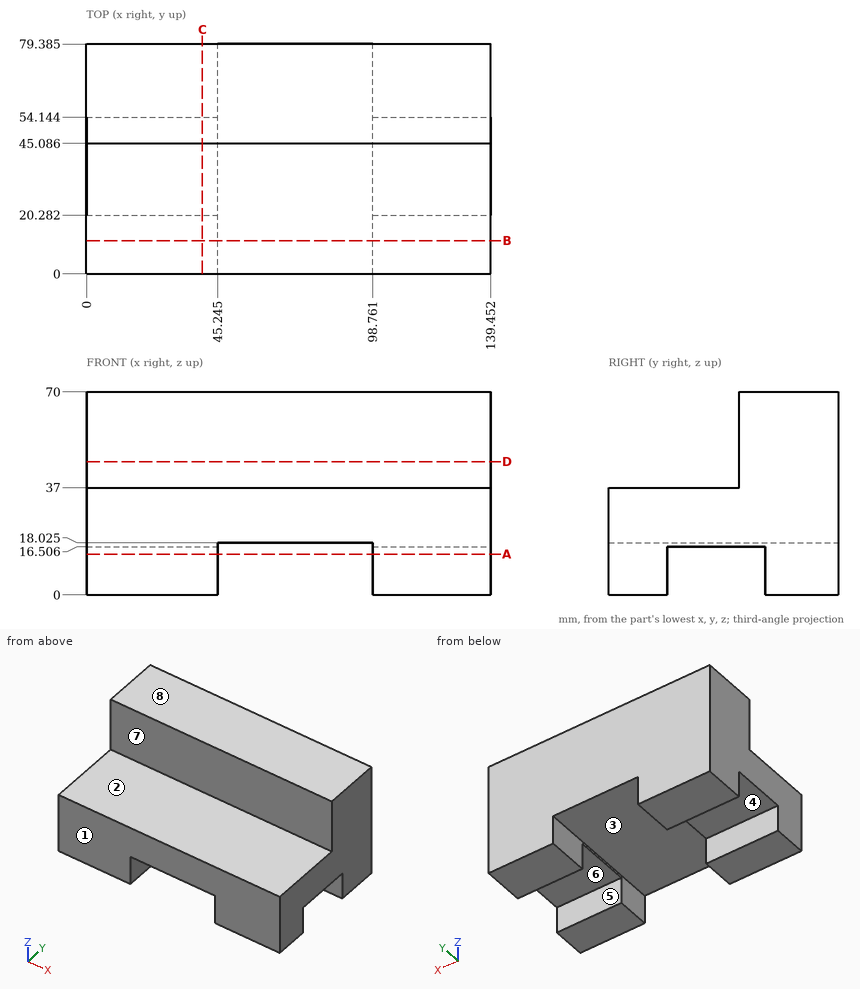
Drawing for the job (mm, zero at the part's lowest x, y, z). A direction names the side the tool comes from. Coordinates: 2 decimals unless noted, no trailing zeros. Write each loop counter-clockwise with the first axis right and the second up, starting at its lowest first coordinate (ties: lowest second). Pieces come first, ordered by that corner, then holes. Notation, with made-up numbers: (79, 51) -> (133, 51) arc R21 ccw to (133, 55) -> close; hole circle Ø5 at (82, 72.25). An arc over 180 degrees is marked (long way). One line per item, written item: value. Start each with the question number.
1) Probe probe 1 along X at (y, z) = (75, 9.5) (1 decimal); probe 2 along Y at (x, z) = (95, 59) (1 decimal); probe 3 along Z at (x, y) = (94, 9) (1 decimal). List the from-to ranges inside material, lowest first.
2) Slice it at B-B on y = 11.5. Write the cut outline in (x, z) (1 decimal).
3) Slice it at C-C on x = 40. Write the cut outline in (y, z) (1 decimal).
4) Pull direction Y, two halves, no side cores. Call the marked faces 5, 6, 7 and 8: +Y half, -Y half, draft (parallel to the pull), parting line (faces both ways), or undercut.
5) Which spindle directions (+Z, -Z, +X, -X, +Y, -Y) get a long thin tool onto all of the face, cutting with end or side? Do the marked faces 1, 2, 3 and 4. Say none if no direction does.
6) Flat gauge pins, fed straight in: pin 1 Ø10 at (x, y) = (122, 35.5) entering from -Z; pin 2 Ø3 at (x, y) = (18, 35.5) entering from +Z; pin 3 Ø6 at (x, y) = (53.5, 70.5) entering from -Z (3 decimals); pin 4 Ø1 at (x, z) = (47, 17) entering from -Y. Where does each tip first touch, or does it go through?
7) Slice it at A-A on z = 14. Write the cut outline in (x, y) (1 decimal).
8) Slice it at D-D on z = 46. Write the cut outline in (x, y) (1 decimal), then the cut area to 3 significant figures.
Answers follow:
1. probe 1: 0 to 45.2, 98.8 to 139.5
1. probe 2: 45.1 to 79.4
1. probe 3: 18 to 37
2. outline: (0, 0) -> (45.2, 0) -> (45.2, 18) -> (98.8, 18) -> (98.8, 0) -> (139.5, 0) -> (139.5, 37) -> (0, 37) -> close
3. outline: (0, 0) -> (20.3, 0) -> (20.3, 16.5) -> (54.1, 16.5) -> (54.1, 0) -> (79.4, 0) -> (79.4, 70) -> (45.1, 70) -> (45.1, 37) -> (0, 37) -> close
4. face 5: undercut
4. face 6: undercut
4. face 7: -Y half
4. face 8: draft
5. face 1: +Z, -Z, +X, -X, -Y
5. face 2: +Z, +X, -X, -Y
5. face 3: -Z, +Y, -Y
5. face 4: -Z, +X, -X
6. pin 1: z = 16.51
6. pin 2: z = 37
6. pin 3: z = 18.025
6. pin 4: through
7. outline: (0, 0) -> (45.2, 0) -> (45.2, 20.3) -> (0, 20.3) -> close; (0, 54.1) -> (45.2, 54.1) -> (45.2, 79.4) -> (0, 79.4) -> close; (98.8, 0) -> (139.5, 0) -> (139.5, 20.3) -> (98.8, 20.3) -> close; (98.8, 54.1) -> (139.5, 54.1) -> (139.5, 79.4) -> (98.8, 79.4) -> close
8. outline: (0, 45.1) -> (139.5, 45.1) -> (139.5, 79.4) -> (0, 79.4) -> close
8. area: 4,780 mm2
